from build123d import *

# Parameters (mm, degrees)
BOSS_EXTRUDE1_DEPTH = 6
SKETCH2_W           = 15
SKETCH2_H           = 192
SKETCH2_H_2         = 236
CUT_EXTRUDE1_DEPTH  = 6
SKETCH3_W           = 114
SKETCH3_H           = 80
CUT_EXTRUDE2_DEPTH  = 6
SKETCH5_W           = 20
SKETCH5_H           = 6
CUT_EXTRUDE5_DEPTH  = 6
SKETCH6_R           = 2.5
CUT_EXTRUDE7_DEPTH  = 6
SKETCH7_W           = 59
SKETCH7_H           = 3.87
CUT_EXTRUDE8_DEPTH  = 6
CUT_EXTRUDE10_DEPTH = 6
SKETCH10_W          = 12
SKETCH10_H          = 6
CUT_EXTRUDE11_DEPTH = 6


with BuildPart() as part:
    # Sketch1 → Boss-Extrude1 (new body)
    with BuildSketch(Plane.XY):
        Polygon((-86, 90.5), (-80, 90.5), (-80, 110.5), (80, 110.5), (80, 90.5), (86, 90.5), (86, 70.5), (80, 70.5), (80, 50.5), (86, 50.5), (86, 30.5), (80, 30.5), (80, 10.5), (86, 10.5), (86, -9.5), (80, -9.5), (80, -29.5), (86, -29.5), (86, -49.5), (80, -49.5), (80, -69.5), (86, -69.5), (86, -89.5), (80, -89.5), (80, -109.5), (86, -109.5), (86, -129.5), (80, -129.5), (80, -149.5), (86, -149.5), (86, -169.5), (80, -169.5), (-86, -169.5), (-86, -30.5), (-80, -30.5), (-80, -9.5), (-86, -9.5), (-86, 10.5), (-80, 10.5), (-80, 30.5), (-86, 30.5), (-86, 50.5), (-80, 50.5), (-80, 70.5), (-86, 70.5), align=None)
    extrude(amount=BOSS_EXTRUDE1_DEPTH)

    # Sketch2 → Cut-Extrude1 (cut)
    with BuildSketch(Plane.XY):
        with Locations((-67.5, -13.5)):
            Rectangle(SKETCH2_W, SKETCH2_H)
        with Locations((67.5, -35.5)):
            Rectangle(SKETCH2_W, SKETCH2_H_2)
    extrude(amount=CUT_EXTRUDE1_DEPTH, mode=Mode.SUBTRACT)

    # Sketch3 → Cut-Extrude2 (cut)
    with BuildSketch(Plane.XY.offset(6)):
        with Locations((0, 42.5)):
            Rectangle(SKETCH3_W, SKETCH3_H)
    extrude(amount=-CUT_EXTRUDE2_DEPTH, mode=Mode.SUBTRACT)

    # Sketch5 → Cut-Extrude5 (cut)
    with BuildSketch(Plane(origin=(0, 0, 0), x_dir=(-1, 0, 0), z_dir=(0, 0, -1))):
        with Locations((40, -0.5)):
            Rectangle(SKETCH5_W, SKETCH5_H)
        with Locations((0, -0.5)):
            Rectangle(SKETCH5_W, SKETCH5_H)
        with Locations((-40, -0.5)):
            Rectangle(SKETCH5_W, SKETCH5_H)
    extrude(amount=-CUT_EXTRUDE5_DEPTH, mode=Mode.SUBTRACT)

    # Sketch6 → Cut-Extrude7 (cut)
    with BuildSketch(Plane.XY.offset(6)):
        with Locations((-80.5, -56.5)):
            Circle(SKETCH6_R)
    extrude(amount=-CUT_EXTRUDE7_DEPTH, mode=Mode.SUBTRACT)

    # Sketch7 → Cut-Extrude8 (cut)
    with BuildSketch(Plane(origin=(0, 0, 0), x_dir=(-1, 0, 0), z_dir=(0, 0, -1))):
        with Locations((0, 108.565)):
            Rectangle(SKETCH7_W, SKETCH7_H)
    extrude(amount=-CUT_EXTRUDE8_DEPTH, mode=Mode.SUBTRACT)

    # Sketch9 → Cut-Extrude10 (cut)
    with BuildSketch(Plane.XY.offset(6)):
        with BuildLine():
            Line((-86, -169.5), (2, -169.5))
            Line((2, -169.5), (2, -124.5))
            ThreePointArc((2, -124.5), (-0.928932188, -117.428932188), (-8, -114.5))
            Line((-8, -114.5), (-86, -114.5))
            Line((-86, -114.5), (-86, -169.5))
        make_face()
    extrude(amount=-CUT_EXTRUDE10_DEPTH, mode=Mode.SUBTRACT)

    # Sketch10 → Cut-Extrude11 (cut)
    with BuildSketch(Plane.XY.offset(6)):
        with Locations((28, -166.5)):
            Rectangle(SKETCH10_W, SKETCH10_H)
        with Locations((60, -166.5)):
            Rectangle(SKETCH10_W, SKETCH10_H)
    extrude(amount=-CUT_EXTRUDE11_DEPTH, mode=Mode.SUBTRACT)


solid = part.part
The listing builds one solid part. Answer for the finished solid, in the listing's coordinates (mm). A direction names the side the tool comes from. Round coordinates to 2 decimals unless told otherwise and drop trailing zeros. Order: outer loops, then holes, each group sorted by start corner. A loop starts at its lowest first (then second) coordinate and runs counter-clockwise, first axis right, second up. Notation, with made-up numbers: (-35.5, 61.25) -> (1.5, 61.25) arc R29 cw to (1.5, 98.25) -> close; hole circle Ø2 at (64, 54.5). An arc over 180 degrees is marked (long way). One line per item, written item: value.
Item 1: Find section B-B, the plane x = 42. Give the vertices of the cut face in (y, z), then the cut area to 3 significant figures.
Taken from the geometry:
outline: (-169.5, 0) -> (-3.5, 0) -> (-3.5, 6) -> (-169.5, 6) -> close; (82.5, 0) -> (110.5, 0) -> (110.5, 6) -> (82.5, 6) -> close
area: 1,160 mm2
Item 2: Given P1, Ø3, axis at x = 82, z = 2.5, coming from the +Y side; P2, Ø1.5, axis at y = -60, z = 1.5, coming from the +X side; P3, Ø3, axis at y = 23, z = 3.5, coming from the -X side, each flat-ended and moving along its own axis, determine where each tip first touches the part or whether it passes through.
Taken from the geometry:
P1: stops at y = 90.5
P2: stops at x = 80
P3: stops at x = -80
Item 3: Find section D-D, the plane z = 2.55. State how many separate pieces and enclosed holes the cut face has, then the cut area to 3 significant figures.
Taken from the geometry:
separate pieces: 1
enclosed holes: 4
area: 25,700 mm2
Item 4: For a pull along X with two mould halves and no side action, classify faces 4 (the flat face through (-1, 82.5, 3)), 5 (the flat face through (-83, 50.5, 3)), 6 (the flat face through (-86, 40, 3)) as released by +X, released by -X, zero draft, split by the parting line, or undercut.
Taken from the geometry:
face 4: undercut
face 5: zero draft
face 6: released by -X
Item 5: For faces 1 (the flat face through (83, -109.5, 3)), 2 (the flat face through (-83, 70.5, 3)), 3 (the flat face through (-10, -1, 3)), determine the directions among +Z, -Z, +X, -X, +Y, -Y from which every point of the face is accessible in a straight line to the end or side of a thin tool.
Taken from the geometry:
face 1: +Z, -Z, +X
face 2: +Z, -Z, -X
face 3: +Z, -Z
Item 6: Straight lines are drawn through the part: L1, parallel to Y at x = -80.5, z = 3.9; L2, parallel to X at y = 28.5, z = 0.4; L3, parallel to X at y = 44, z = 4.1. For each, find the intervals that lie inside material, in ascending order.
Taken from the geometry:
L1: y = -114.5 to -59, -54 to -30.5, -9.5 to 10.5, 30.5 to 50.5, 70.5 to 90.5
L2: x = -80 to -75, -60 to -57, 57 to 60, 75 to 80
L3: x = -86 to -75, -60 to -57, 57 to 60, 75 to 86
Item 7: Find section C-C, the plane y = -92.5. Give the vertices of the cut face in (x, z).
Taken from the geometry:
outline: (-86, 0) -> (-75, 0) -> (-75, 6) -> (-86, 6) -> close; (-60, 0) -> (60, 0) -> (60, 6) -> (-60, 6) -> close; (75, 0) -> (80, 0) -> (80, 6) -> (75, 6) -> close
Item 8: Find section A-A, the plane y = -19. Give the vertices of the cut face in (x, z), then the cut area to 3 significant figures.
Taken from the geometry:
outline: (-80, 0) -> (-75, 0) -> (-75, 6) -> (-80, 6) -> close; (-60, 0) -> (60, 0) -> (60, 6) -> (-60, 6) -> close; (75, 0) -> (80, 0) -> (80, 6) -> (75, 6) -> close
area: 780 mm2
